from build123d import *
from OCP.BRepFilletAPI import BRepFilletAPI_MakeChamfer

# Parameters (mm, degrees)
SKETCH1_W           = 60.96
SKETCH1_H           = 16.51
SKETCH1_W_2         = 50.8
SKETCH1_H_2         = 6.35
BOSS_EXTRUDE1_DEPTH = 19.05
BOSS_EXTRUDE2_DEPTH = 16.51
SKETCH5_R           = 1.524
CUT_EXTRUDE1_DEPTH  = 96.537432978
CHAMFER1_SIZE       = 2.1082
CHAMFER1_SIZE2      = 1.832630301
FILLET1_R           = 18.034
CHAMFER2_SIZE       = 2.54
CHAMFER2_SIZE2      = 2.207988314
SKETCH6_W           = 52.07
SKETCH6_H           = 7.62
CUT_EXTRUDE2_DEPTH  = 19.05
SKETCH7_W           = 7.62
SKETCH7_H           = 52.07
CUT_EXTRUDE3_DEPTH  = 19.05


with BuildPart() as part:
    # Sketch1 → Boss-Extrude1 (new body)
    with BuildSketch(Plane(origin=(0, 0, 0), x_dir=(1, 0, 0), z_dir=(0, 1, 0))):
        Rectangle(SKETCH1_W, SKETCH1_H)
        Rectangle(SKETCH1_W_2, SKETCH1_H_2, mode=Mode.SUBTRACT)
    boss_extrude1 = extrude(amount=BOSS_EXTRUDE1_DEPTH)

    # Sketch2 → Boss-Extrude2 (add)
    with BuildSketch(Plane.XY.offset(8.255)):
        with BuildLine():
            Line((-30.48, 19.05), (-30.48, 80.01))
            ThreePointArc((-30.48, 80.01), (12.625229381, 62.155229381), (30.48, 19.05))
            Line((30.48, 19.05), (-30.48, 19.05))
        make_face()
    extrude(amount=-BOSS_EXTRUDE2_DEPTH)

    # Mirror1: Boss-Extrude1 across plane
    add(boss_extrude1.mirror(Plane(origin=(-24.765, 24.765, 0), x_dir=(0, 0, 1), z_dir=(-0.7071067811865488, 0.7071067811865464, 0))))

    # Sketch5 → Cut-Extrude1 (cut, through all)
    with BuildSketch(Plane(origin=(0, 0, -8.255), x_dir=(-1, 0, 0), z_dir=(0, 0, -1))):
        with Locations((0, 9.917240348)):
            Circle(SKETCH5_R)
        with Locations((39.468758027, 49.53)):
            Circle(SKETCH5_R)
        with BuildLine():
            Line((-2.778172553, 66.109095279), (-28.061671506, 36.049832271))
            ThreePointArc((-28.061671506, 36.049832271), (-10.480017479, 64.198627533), (19.242304668, 78.965238493))
            ThreePointArc((19.242304668, 78.965238493), (7.11859344, 74.444363935), (-2.778172553, 66.109095279))
        make_face()
    extrude(amount=-CUT_EXTRUDE1_DEPTH, mode=Mode.SUBTRACT)

    # Chamfer1
    chamfer1_edges = [part.edges().sort_by_distance(p)[0] for p in [
        (1.524, 9.917240348, -8.255),
        (-37.944758027, 49.53, -8.255),
    ]]
    chamfer1_side = [part.faces().sort_by_distance(p)[0] for p in [
        (-12.284487688, 37.419339753, -8.255),
    ]]
    chamfer(chamfer1_edges, length=CHAMFER1_SIZE, length2=CHAMFER1_SIZE2, reference=chamfer1_side[0])

    # Fillet1
    fillet1_edges = [part.edges().sort_by_distance(p)[0] for p in [
        (28.061671506, 36.049832271, 0),
    ]]
    fillet(fillet1_edges, radius=FILLET1_R)

    # Chamfer2: one chamfer whose edges measure the first distance from different faces: ONE call of the kernel's chamfer builder (chamfer() names one face for all edges)
    chamfer2_edges_1 = [part.edges().sort_by_distance(p)[0] for p in [
        (14.079711572, 52.672824674, 8.255),
    ]]
    chamfer2_side_1 = [part.faces().sort_by_distance(p)[0] for p in [
        (14.079711572, 52.672824674, 0),
    ]]
    chamfer2_edges_2 = [part.edges().sort_by_distance(p)[0] for p in [
        (27.816828301, 35.476442899, 8.255),
    ]]
    chamfer2_side_2 = [part.faces().sort_by_distance(p)[0] for p in [
        (27.816828301, 35.476442899, 0),
    ]]
    chamfer2_edges_3 = [part.edges().sort_by_distance(p)[0] for p in [
        (30.171820892, 25.171945968, 8.255),
    ]]
    chamfer2_side_3 = [part.faces().sort_by_distance(p)[0] for p in [
        (30.171820892, 25.171945968, 0),
    ]]
    chamfer2_edges_4 = [part.edges().sort_by_distance(p)[0] for p in [
        (-40.005, 80.01, 8.255),
    ]]
    chamfer2_side_4 = [part.faces().sort_by_distance(p)[0] for p in [
        (-40.005, 80.01, 0),
    ]]
    chamfer2_edges_5 = [part.edges().sort_by_distance(p)[0] for p in [
        (30.48, 9.525, 8.255),
    ]]
    chamfer2_side_5 = [part.faces().sort_by_distance(p)[0] for p in [
        (30.48, 9.525, 0),
    ]]
    chamfer2_edges_6 = [part.edges().sort_by_distance(p)[0] for p in [
        (-24.836921873, 79.748247662, 8.255),
    ]]
    chamfer2_side_6 = [part.faces().sort_by_distance(p)[0] for p in [
        (-24.836921873, 79.748247662, 0),
    ]]
    chamfer2_edges_7 = [part.edges().sort_by_distance(p)[0] for p in [
        (-7.11859344, 74.444363935, 8.255),
    ]]
    chamfer2_side_7 = [part.faces().sort_by_distance(p)[0] for p in [
        (-7.11859344, 74.444363935, 0),
    ]]
    chamfer2 = BRepFilletAPI_MakeChamfer(part.part.solid().wrapped)
    for e in chamfer2_edges_1:
        chamfer2.Add(CHAMFER2_SIZE, CHAMFER2_SIZE2, e.wrapped, chamfer2_side_1[0].wrapped)  # the first distance lies on this face
    for e in chamfer2_edges_2:
        chamfer2.Add(CHAMFER2_SIZE, CHAMFER2_SIZE2, e.wrapped, chamfer2_side_2[0].wrapped)  # the first distance lies on this face
    for e in chamfer2_edges_3:
        chamfer2.Add(CHAMFER2_SIZE, CHAMFER2_SIZE2, e.wrapped, chamfer2_side_3[0].wrapped)  # the first distance lies on this face
    for e in chamfer2_edges_4:
        chamfer2.Add(CHAMFER2_SIZE, CHAMFER2_SIZE2, e.wrapped, chamfer2_side_4[0].wrapped)  # the first distance lies on this face
    for e in chamfer2_edges_5:
        chamfer2.Add(CHAMFER2_SIZE, CHAMFER2_SIZE2, e.wrapped, chamfer2_side_5[0].wrapped)  # the first distance lies on this face
    for e in chamfer2_edges_6:
        chamfer2.Add(CHAMFER2_SIZE, CHAMFER2_SIZE2, e.wrapped, chamfer2_side_6[0].wrapped)  # the first distance lies on this face
    for e in chamfer2_edges_7:
        chamfer2.Add(CHAMFER2_SIZE, CHAMFER2_SIZE2, e.wrapped, chamfer2_side_7[0].wrapped)  # the first distance lies on this face
    add(Compound.cast(chamfer2.Shape()), mode=Mode.REPLACE)

    # Sketch6 → Cut-Extrude2 (cut)
    with BuildSketch(Plane.XZ):
        Rectangle(SKETCH6_W, SKETCH6_H)
    extrude(amount=-CUT_EXTRUDE2_DEPTH, mode=Mode.SUBTRACT)

    # Sketch7 → Cut-Extrude3 (cut)
    with BuildSketch(Plane.ZY.offset(49.53)):
        with Locations((0, 49.53)):
            Rectangle(SKETCH7_W, SKETCH7_H)
    extrude(amount=-CUT_EXTRUDE3_DEPTH, mode=Mode.SUBTRACT)


solid = part.part
Could you check a few things on this model? Use its own coordinates, in mm. A direction names the side the tool comes from. Give positions to 0.01 mm unless a question says otherwise; leave off trailing zeros. Order: outer loops, then holes, each group sorted by start corner. A loop starts at its lowest first (then second) coordinate and runs counter-clockwise, first axis right, second up.
1. Suppose I cut it at D-D (z = 6.75). List the corners of the cut face in (x, y) for me.
2. Suppose I cut it at C-C (x = 19.5). List the corners of the cut face in (y, z) for me (3 decimals), plus the area to 3 significant figures.
3. For faces 5 (the cylindrical face through (30.163, 25.257, -1.172)), 6 (the flat face through (-30.48, 9, 0)), 7 (the flat face through (0, 12, 3.81)), which set-ups out of +Z, -Z, +X, -X, +Y, -Y let a thin tool reach every point of the face, with its end or its side?
4. I need wall thicknesses on L1, parallel to X at y = 15, z = -3.5 (3 decimals); L2, parallel to Y at x = -31, z = 1 (3 decimals); L3, parallel to Z at x = -25, y = 13 (3 decimals). Which ranges of each line are inside material? Lowest first, please.
5. We'd pull the mould along Y, two halves only. Please class faces 1 (the flat face through (-40, 23.495, 0)), 2 (the flat face through (-26.035, 9, 0)), 3 (the cylindrical face through (-7.28, 74.54, -1.37)), 4 (the cylindrical face through (-40.92, 49.99, 6)): pulls with the +Y half, pulls with the -Y half, needs draft (parallel to the pull), parting line crosses it, or undercut.
6. Suppose I cut it at A-A (z = 2.5). List the corners of the cut face in (x, y) for me (3 decimals), plus the area to 3 significant figures.
7. Suppose I cut it at B-B (y = 49.53). List the corners of the cut face in (x, z) for me (3 decimals), plus the area to 3 significant figures.
8. Will these pins go through, and if not, where does the flat tip stop? P1, Ø4, axis at y = 38, z = 1.5, coming from the +X side; P2, Ø2.5, axis at x = 0, y = 9.92, coming from the -Z side; P3, Ø4, axis at x = 0, y = 9.92, coming from the +Z side (3 decimals); P4, Ø2, axis at y = 37.5, z = 2.5, coming from the -X side.
Solved:
1. outline: (-49.53, 19.05) - (-30.48, 19.05) - (-30.48, 0) - (29.58, 0) - (29.58, 19.05) arc R60.06 ccw to (28.37, 31.05) arc R17.13 ccw to (24.69, 38.66) - (2.09, 65.53) arc R37.01 ccw to (-19.41, 78.08) arc R60.06 ccw to (-30.48, 79.11) - (-49.53, 79.11) - close; hole circle Ø3.05 at (-39.47, 49.53); hole circle Ø3.05 at (0, 9.92)
2. outline: (0, -8.255) - (46.229, -8.255) - (46.229, 5.715) - (42.799, 8.255) - (0, 8.255) - (0, 3.81) - (19.05, 3.81) - (19.05, -3.81) - (0, -3.81) - close
2. area: 614 mm2
3. face 5: +Z, -Z, +X, +Y
3. face 6: +Z, -Z, -X, -Y
3. face 7: -Y
4. L1: x = -30.48 to -26.035, 26.035 to 30.48
4. L2: y = 19.05 to 23.495, 75.565 to 80.01
4. L3: z = -8.255 to -3.81, 3.81 to 8.255
5. face 1: undercut
5. face 2: needs draft
5. face 3: pulls with the +Y half
5. face 4: undercut
6. outline: (-49.53, 19.05) - (-30.48, 19.05) - (-30.48, 0) - (-26.035, 0) - (-26.035, 19.05) - (26.035, 19.05) - (26.035, 0) - (30.48, 0) - (30.48, 19.05) arc R60.96 ccw to (29.25, 31.232) arc R18.034 ccw to (25.381, 39.237) - (2.778, 66.109) arc R37.905 ccw to (-19.242, 78.965) arc R60.96 ccw to (-30.48, 80.01) - (-49.53, 80.01) - (-49.53, 75.565) - (-30.48, 75.565) - (-30.48, 23.495) - (-49.53, 23.495) - close
6. area: 3,070 mm2
7. outline: (-49.53, -8.255) - (-43.101, -8.255) - (-40.993, -6.422) - (-40.993, -3.81) - (-49.53, -3.81) - close; (-49.53, 3.81) - (-40.993, 3.81) - (-40.993, 8.255) - (-49.53, 8.255) - close; (-37.945, -6.422) - (-35.837, -8.255) - (16.723, -8.255) - (16.723, 5.715) - (13.838, 8.255) - (-37.945, 8.255) - (-37.945, 3.81) - (-30.48, 3.81) - (-30.48, -3.81) - (-37.945, -3.81) - close
7. area: 914 mm2
8. P1: stops at x = 27.55
8. P2: passes through
8. P3: stops at z = 8.255
8. P4: stops at x = -30.48
